```python
from build123d import *

# Parameters (mm, degrees)
EXTRUDE_1_DEPTH     = 2.5
SKETCH_3_R          = 2.5
CUT_EXTRUDE_2_DEPTH = 8
SKETCH_5_R          = 2.5
CUT_EXTRUDE_4_DEPTH = 8


with BuildPart() as part:
    # 草图1 → 凸台-拉伸1 (new, symmetric)
    with BuildSketch(Plane.XY):
        with BuildLine():
            Line((-69.221317243, 27.986194726), (0.778682757, 27.986194726))
            ThreePointArc((0.778682757, 27.986194726), (5.778682757, 22.986194726), (0.778682757, 17.986194726))
            Line((0.778682757, 17.986194726), (-69.221317243, 17.986194726))
            ThreePointArc((-69.221317243, 17.986194726), (-74.221317243, 22.986194726), (-69.221317243, 27.986194726))
        make_face()
    extrude(amount=EXTRUDE_1_DEPTH, both=True)

    # 草图3 → 切除-拉伸2 (cut)
    with BuildSketch(Plane.XY.offset(2.5)):
        with Locations((-69.221317243, 22.986194726)):
            Circle(SKETCH_3_R)
    extrude(amount=-CUT_EXTRUDE_2_DEPTH, mode=Mode.SUBTRACT)

    # 草图5 → 切除-拉伸4 (cut)
    with BuildSketch(Plane.XY.offset(2.5)):
        with Locations((0.778682757, 22.986194726)):
            Circle(SKETCH_5_R)
    extrude(amount=-CUT_EXTRUDE_4_DEPTH, mode=Mode.SUBTRACT)


solid = part.part
```
Geometry check sheet. Reference: the model listing, model coordinates, mm. Round coordinates to 2 decimals unless told otherwise and drop trailing zeros. Loops run counter-clockwise (first coordinate to the right, second up) from the corner with the lowest first, then second, coordinate; pieces in that order, holes last. Notation, with made-up numbers: M 13,6 L 42,6 A23 cw 42,45 Z; hole C -6.5,89.5 d7. An arc over 180 degrees is marked long. Return JSON: item names as keys, results as strings. Group by question number.
(1) Section check B-B, the plane z = -0.25. Enter the section's corners in (x, y).
(2) Section check C-C, the plane y = 27. Enter the section's corners in (x, z).
(3) Mould release check, pull along Y, two halves, no side actions. Record for faces 1 (the face through (2.123, 25.094, 0.035)), 2 (the face through (-74.22, 22.88, 0.04)), 3 (the face through (-34, 17.986, 0)), 4 (the face through (-71.72, 23.1, 0.04)): pulls with the +Y half, pulls with the -Y half, needs draft (parallel to the pull), parting line crosses it, or undercut.
(4) Section check A-A, the plane y = 21.5. Enter the section's corners in (x, z).
(5) Go/stop test with a flat-tipped pin: pin 1 (2 mm diameter, centred on y = 21.5, z = 1.5, fed in from -X). Record where the tip stops, or that it passes through.
(6) Scan lines: line 1 along X through (y, z) = (22.75, -2.3); line 2 along X through (y, z) = (24.75, 1); line 3 along Y through (x, z) = (-67, -0.95). Record each from-to range of solid material in increasing order. Write a range as [from, to].
Data:
{
 "1": {"outline": "M -69.22,17.99 L 0.78,17.99 A5 ccw 0.78,27.99 L -69.22,27.99 A5 ccw Z; hole C -69.22,22.99 d5; hole C 0.78,22.99 d5"},
 "2": {"outline": "M -72.2,-2.5 L 3.76,-2.5 L 3.76,2.5 L -72.2,2.5 Z"},
 "3": {"face 1": "undercut", "face 2": "parting line crosses it", "face 3": "pulls with the -Y half", "face 4": "undercut"},
 "4": {"outline": "M -74,-2.5 L -71.23,-2.5 L -71.23,2.5 L -74,2.5 Z; M -67.21,-2.5 L -1.23,-2.5 L -1.23,2.5 L -67.21,2.5 Z; M 2.79,-2.5 L 5.55,-2.5 L 5.55,2.5 L 2.79,2.5 Z"},
 "5": {"pin 1": "x = -74.2"},
 "6": {"line 1": "[-74.22, -71.71], [-66.73, -1.71], [3.27, 5.77]", "line 2": "[-73.9, -70.99], [-67.45, -0.99], [2.55, 5.46]", "line 3": "[17.99, 21.84], [24.13, 27.99]"}
}
